from build123d import *

# Parameters (mm, degrees)
SKETCH1_W                               = 150
SKETCH1_H                               = 60
BOSS_EXTRUDE1_DEPTH                     = 10
CBORE_FOR_M5_HEX_HEAD_BOLT1_D           = 5.5
CBORE_FOR_M5_HEX_HEAD_BOLT1_CBORE_D     = 12.238
CBORE_FOR_M5_HEX_HEAD_BOLT1_CBORE_DEPTH = 3.5
SKETCH4_W                               = 32
SKETCH4_H                               = 40
BOSS_EXTRUDE2_DEPTH                     = 120
CUT_EXTRUDE1_DEPTH                      = 120
BOSS_EXTRUDE3_DEPTH                     = 42.720018727
CUT_EXTRUDE2_DEPTH                      = 45.625
SKETCH10_W                              = 17
SKETCH10_H                              = 10
BOSS_EXTRUDE4_DEPTH                     = 120
SKETCH11_W                              = 17
SKETCH11_H                              = 14
BOSS_EXTRUDE5_DEPTH                     = 80
CUT_EXTRUDE3_DEPTH                      = 95
FILLET1_R                               = 5
FILLET2_R                               = 5
FILLET3_R                               = 5
FILLET4_R                               = 1


with BuildPart() as part:
    # Sketch1 → Boss-Extrude1 (new body)
    with BuildSketch(Plane.XY):
        Rectangle(SKETCH1_W, SKETCH1_H)
    extrude(amount=BOSS_EXTRUDE1_DEPTH)

    # CBORE for M5 Hex Head Bolt1 (through all)
    with Locations(Plane(origin=(-55, 0, 10), x_dir=(1, 0, 0), z_dir=(0, 0, 1))):
        with Locations((0, 0), (110, 0)):
            CounterBoreHole(CBORE_FOR_M5_HEX_HEAD_BOLT1_D / 2, CBORE_FOR_M5_HEX_HEAD_BOLT1_CBORE_D / 2, CBORE_FOR_M5_HEX_HEAD_BOLT1_CBORE_DEPTH)

    # Sketch4 → Boss-Extrude2 (add)
    with BuildSketch(Plane.XY.offset(10)):
        Rectangle(SKETCH4_W, SKETCH4_H)
    extrude(amount=BOSS_EXTRUDE2_DEPTH)

    # Sketch7 → Cut-Extrude1 (cut)
    with BuildSketch(Plane(origin=(16, 0, 0), x_dir=(0, 0, -1), z_dir=(1, 0, 0))):
        Polygon((-130, 20), (-115, -20), (-130, -20), align=None)
    extrude(amount=-CUT_EXTRUDE1_DEPTH, mode=Mode.SUBTRACT)

    # Sketch8 → Boss-Extrude3 (add, along a direction that is not the sketch's normal)
    with BuildSketch(Plane(origin=(0, 20, 0), x_dir=(1, 0, 0), z_dir=(0, 1, 0))):
        with BuildLine():
            Line((-16, -130), (16, -130))
            ThreePointArc((16, -130), (0, -146), (-16, -130))
        make_face()
    extrude(amount=-BOSS_EXTRUDE3_DEPTH, dir=(0, 0.9363291775690444, 0.351123441588392))

    # Sketch9 → Cut-Extrude2 (cut, along a direction that is not the sketch's normal)
    with BuildSketch(Plane(origin=(0, 20, 0), x_dir=(1, 0, 0), z_dir=(0, 1, 0))):
        with BuildLine():
            Line((8.5, -94), (8.5, -130))
            ThreePointArc((8.5, -130), (0, -138.5), (-8.5, -130))
            Line((-8.5, -130), (-8.5, -94))
            ThreePointArc((-8.5, -94), (0, -85.5), (8.5, -94))
        make_face()
    extrude(amount=-CUT_EXTRUDE2_DEPTH, dir=(0, 0.9363291775690444, 0.351123441588392), mode=Mode.SUBTRACT)

    # Sketch10 → Boss-Extrude4 (add)
    with BuildSketch(Plane(origin=(0, 30, 0), x_dir=(1, 0, 0), z_dir=(0, 1, 0))):
        with Locations((0, -5)):
            Rectangle(SKETCH10_W, SKETCH10_H)
    extrude(amount=BOSS_EXTRUDE4_DEPTH)

    # Sketch11 → Boss-Extrude5 (add)
    with BuildSketch(Plane.XY.offset(10)):
        with Locations((0, 143)):
            Rectangle(SKETCH11_W, SKETCH11_H)
    extrude(amount=BOSS_EXTRUDE5_DEPTH)

    # Sketch13 → Cut-Extrude3 (cut)
    with BuildSketch(Plane(origin=(8.5, 0, 0), x_dir=(0, 0, -1), z_dir=(1, 0, 0))):
        Polygon((-85, 143.5), (-85, 138.309401077), (-81, 136), (-73, 136), (-73, 143.5), align=None)
    extrude(amount=-CUT_EXTRUDE3_DEPTH, mode=Mode.SUBTRACT)

    # Fillet1
    fillet1_edges = [part.edges().sort_by_distance(p)[0] for p in [
        (0, 136, 10),
    ]]
    fillet(fillet1_edges, radius=FILLET1_R)

    # Fillet2
    fillet2_edges = [part.edges().sort_by_distance(p)[0] for p in [
        (75, -30, 5),
        (-75, -30, 5),
        (-75, 30, 5),
        (75, 30, 5),
    ]]
    fillet(fillet2_edges, radius=FILLET2_R)

    # Fillet3
    fillet3_edges = [part.edges().sort_by_distance(p)[0] for p in [
        (16, 0, 10),
        (-16, 0, 10),
    ]]
    fillet(fillet3_edges, radius=FILLET3_R)

    # Fillet4
    fillet4_edges = [part.edges().sort_by_distance(p)[0] for p in [
        (0, 143.5, 73),
    ]]
    fillet(fillet4_edges, radius=FILLET4_R)


solid = part.part
Part model, mm, in its own coordinate system. A direction names the side the tool comes from. Coordinates: 2 decimals unless noted, no trailing zeros. Write each loop counter-clockwise with the first axis right and the second up, starting at its lowest first coordinate (ties: lowest second). Pieces come first, ordered by that corner, then holes. Notation, with made-up numbers: (34, 14) - (76, 14) arc R8 cw to (76, 22) - close; hole circle Ø10 at (-29, -37.5). An arc over 180 degrees is marked (long way). Put each result on its own line as item: value.
1. Band-saw the part on C-C (y = 0). Give the number of separate pieces and of enclosed holes in the cut face, then the cut area to 3 significant figures.
Final values:
separate pieces: 3
enclosed holes: 1
area: 4,520 mm²
2. Flat gauge pins, fed straight in: pin 1 Ø3 at (x, z) = (-40, 5.5) entering from +Y; pin 2 Ø4 at (x, z) = (2, 60.5) entering from -Y; pin 3 Ø20 at (y, z) = (5, 114.5) entering from -X; pin 4 Ø4 at (x, y) = (0, 142) entering from -Z. Where does each tip first touch, or does it go through?
Final values:
pin 1: stops at y = 30
pin 2: stops at y = -20
pin 3: stops at x = -16
pin 4: stops at z = 0
3. 3-axis set-ups, long thin cutter, end or side, ignore diameter. For faces 1 (the flat face through (16, 0, 72)), 2 (the cylindrical face through (60.836, 1.838, 8.274)), 3 (the flat face through (0, 136, 44)), 4 (the flat face through (0, 143.5, 79)): which of +Z, -Z, +X, -X, +Y, -Y reach the whole face in a straight line?
Final values:
face 1: +Z, +X, +Y, -Y
face 2: +Z
face 3: +Z, +X, -X
face 4: +X, -X
4. Band-saw the part on D-D (z = 62.5). Write the cut outline in (x, y), then the cut area to 3 significant figures.
Final values:
outline: (-16, -20) - (16, -20) - (16, 20) - (-16, 20) - close; (-8.5, 136) - (8.5, 136) - (8.5, 150) - (-8.5, 150) - close
area: 1,520 mm²
5. Band-saw the part on B-B (x = 55.5). Write the cut outline in (y, z).
Final values:
outline: (-30, 0) - (-2.7, 0) - (-2.7, 6.5) - (-6.1, 6.5) - (-6.1, 10) - (-30, 10) - close; (2.7, 0) - (30, 0) - (30, 10) - (6.1, 10) - (6.1, 6.5) - (2.7, 6.5) - close
6. Two-plate mould, pull along X, no slides. Class faces 5 (the flat face through (8.5, 107, 8)), 6 (the cylindrical face through (-52.253, 0.121, 3.204)), 7 (the flat face through (-16, 0, 72)): +X half, -X half, draft (parallel to the pull), parting line (faces both ways), or undercut.
Final values:
face 5: +X half
face 6: undercut
face 7: -X half
7. Band-saw the part on A-A (z = 103.5). Write the cut outline in (x, y).
Final values:
outline: (-16, -20) - (-8.5, -20) - (-8.5, 20) - (-16, 20) - close; (8.5, -20) - (16, -20) - (16, 20) - (8.5, 20) - close
8. Probe line 1 along Y through (x, z) = (-55, 4); line 2 along X through (y, z) = (-8, 109); line 3 along Y through (x, z) = (-55, 9.1). List the from-to ranges inside material, lowest first. Write a range as [from, to].
Final values:
line 1: y = [-30, -2.75], [2.75, 30]
line 2: x = [-16, -8.5], [8.5, 16]
line 3: y = [-30, -6.12], [6.12, 30]
